Can you work these out from the drawing? Everything is in mm from the part's minimum corner. Round coordinates to 2 decimals unless told otherwise and drop trailing zeros. Use one line per item in the form item = value. Start each with the question number.
Q1. I need wall thicknesses on line 1 along Z through (x, y) = (25.4, 14) (1 decimal); line 2 along Z through (x, y) = (101.6, 8) (1 decimal); line 3 along X through (y, z) = (13.25, 36.5). Which ranges of each line are inside material? Lowest first, please. Write a range as from..to.
Q2. I want a section at A-A on z = 38.1. State how many separate pieces and enclosed holes the cut face has, and give its area (3 significant figures).
Q3. I'm going to push flat-ended pins straight in: pin 1 Ø3 at (x, y) = (101.6, 9.525) entering from -Z; pin 2 Ø5.5 at (x, z) = (101.6, 101.6) entering from +Y. Where does each tip first touch, or does it pass through?
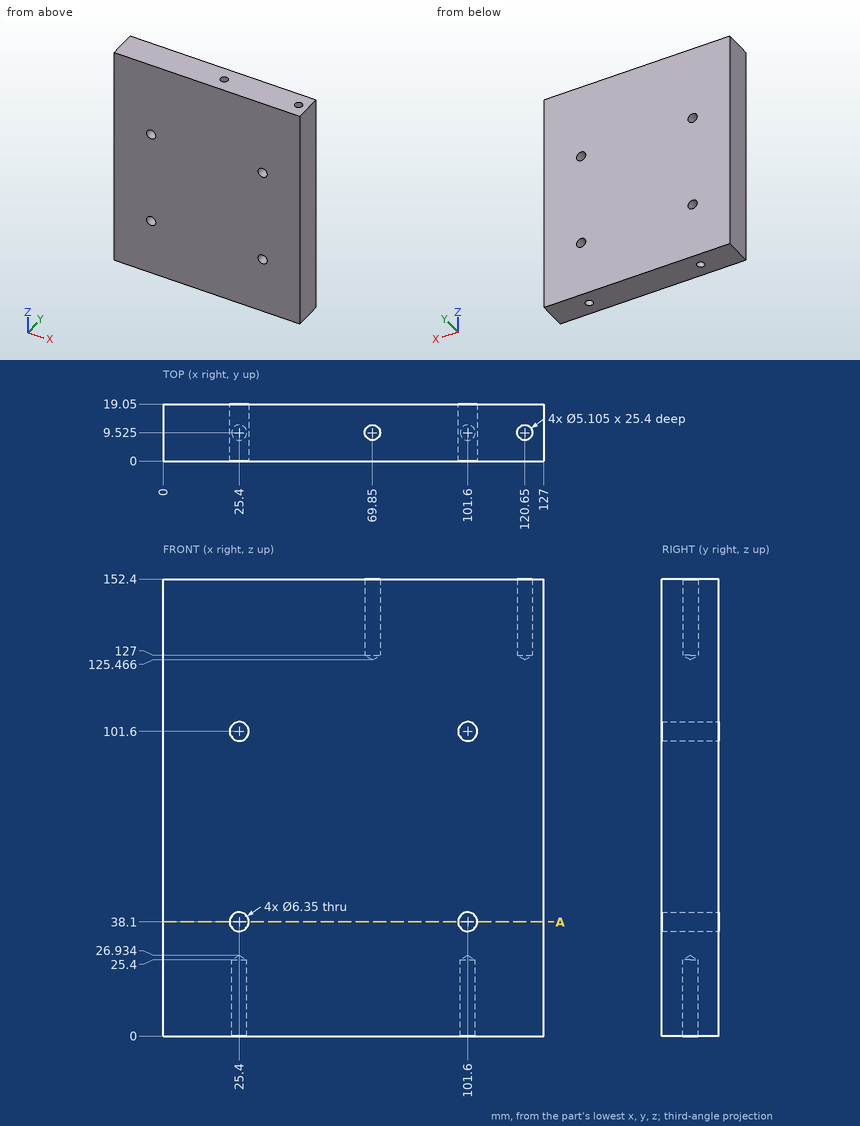
Reported:
q1.line_1 = 0..34.9, 41.3..98.4, 104.8..152.4
q1.line_2 = 26..34.9, 41.3..98.4, 104.8..152.4
q1.line_3 = 0..22.66, 28.14..98.86, 104.34..127
q2.separate_pieces = 3
q2.enclosed_holes = 0
q2.area = 2,180 mm^2
q3.pin_1 = 26.03
q3.pin_2 = through
